Autodesk Inventor part; units mm, degrees
ref_plane "YZ Plane" through (0, 0, 0) normal (1, 0, 0) x (0, 1, 0)
ref_plane "XZ Plane" through (0, 0, 0) normal (0, 1, 0) x (-1, 0, 0)
ref_plane "XY Plane" through (0, 0, 0) normal (0, 0, 1) x (1, 0, 0)
sketch "Sketch1" plane through (0, 0, 0) normal (0, 1, 0) x (-1, 0, 0)
  line L0 (3.7114, 5.7847) -> (-16.2886, 5.7847)
  line L1 (-16.2886, 5.7847) -> (-16.2886, -14.2153)
  line L2 (-16.2886, -14.2153) -> (3.7114, -14.2153)
  line L3 (3.7114, -14.2153) -> (3.7114, 5.7847)
  line L4 (4.2114, 6.2847) -> (-16.7886, 6.2847)
  line L5 (-16.7886, 6.2847) -> (-16.7886, -14.7153)
  line L6 (-16.7886, -14.7153) -> (4.2114, -14.7153)
  line L7 (4.2114, -14.7153) -> (4.2114, 6.2847)
  point P0 (0, 0)
  dimension "d0" = 20
  dimension "d1" = 20
  dimension "d2" = 0.5
extrude "Extrusion2" add sketch "Sketch1" along normal blind 10
For this review, take the finished solid that the model builds, in its own axes (mm). A direction names the side the tool comes from. Round coordinates to 2 decimals unless told otherwise and drop trailing zeros. Order: outer loops, then holes, each group sorted by start corner. A loop starts at its lowest first (then second) coordinate and runs counter-clockwise, first axis right, second up. Notation, with made-up numbers: (43, 28) -> (76, 28) arc R23 cw to (76, 65) -> close; hole circle Ø5 at (-6.75, 61). An arc over 180 degrees is marked (long way). Write item = value, one per line. Start each with the question number.
1) To check wall thickness, follow line 1 (Z direction, x = 6, y = 1.75); line 2 (X direction, y = 2.25, z = 5.25). State the ranges of each line that lie inside material, in increasing order. Write a range as from..to.
2) Take a section at A-A on x = 7.5. State the section outline as (y, z) points.
3) The part is to be moulded in two halves that separate along X. For faces 1 (the face through (16.45, 10, -4.17)), 2 (the face through (6, 5, 5.785)), 3 (the face through (6, 5, -14.215)), 4 (the face through (-4.211, 5, -4)), say which applies: +X half, -X half, draft (parallel to the pull), parting line (faces both ways), or undercut.
4) Tool access review of faces 5 (the face through (16.789, 5, -4)), 6 (the face through (-3.711, 5, -4)): name each direction out of +Z, -Z, +X, -X, +Y, -Y from which nothing blocks a thin tool from reaching the whole face with its end or side.
5) Take a section at B-B on z = -12. State the section outline as (x, y) points.
6) Take a section at C-C on y = 2.5. State the section outline as (x, z) points.
Verdict:
q1.line_1 = -14.72..-14.22, 5.78..6.28
q1.line_2 = -4.21..-3.71, 16.29..16.79
q2.outline = (0, -14.72) -> (10, -14.72) -> (10, -14.22) -> (0, -14.22) -> close; (0, 5.78) -> (10, 5.78) -> (10, 6.28) -> (0, 6.28) -> close
q3.face_1 = draft
q3.face_2 = undercut
q3.face_3 = undercut
q3.face_4 = -X half
q4.face_5 = +Z, -Z, +X, +Y, -Y
q4.face_6 = +Y, -Y
q5.outline = (-4.21, 0) -> (-3.71, 0) -> (-3.71, 10) -> (-4.21, 10) -> close; (16.29, 0) -> (16.79, 0) -> (16.79, 10) -> (16.29, 10) -> close
q6.outline = (-4.21, -14.72) -> (16.79, -14.72) -> (16.79, 6.28) -> (-4.21, 6.28) -> close; hole (-3.71, -14.22) -> (16.29, -14.22) -> (16.29, 5.78) -> (-3.71, 5.78) -> close
